Here's how the part is built. I have some questions about the finished solid (model axes, mm). Face numbers are marked on the shaded views. A direction names the side the tool comes from. Coordinates: 2 decimals unless noted, no trailing zeros. Order: outer loops, then holes, each group sorted by start corner. A loop starts at its lowest first (then second) coordinate and runs counter-clockwise, first axis right, second up.
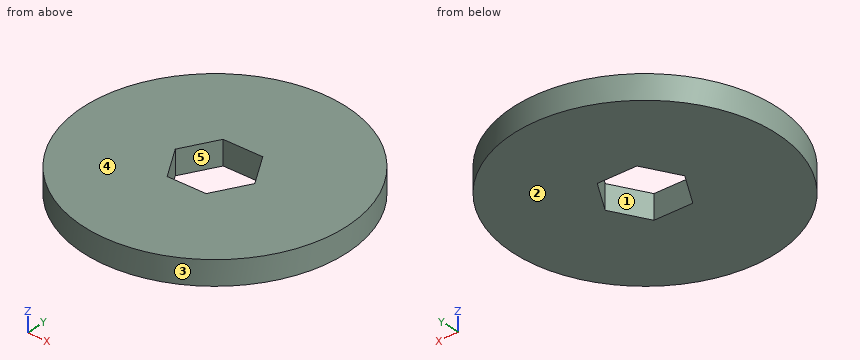
Autodesk Inventor part; units mm, degrees
ref_plane "YZ Plane" through (0, 0, 0) normal (1, 0, 0) x (0, 1, 0)
ref_plane "XZ Plane" through (0, 0, 0) normal (0, 1, 0) x (-1, 0, 0)
ref_plane "XY Plane" through (0, 0, 0) normal (0, 0, 1) x (1, 0, 0)
sketch "Sketch1" plane through (0, 0, 0) normal (0, 0, 1) x (1, 0, 0)
  line L0 (3.6662, 6.35) -> (7.3323, 0)
  line L1 (7.3323, 0) -> (3.6662, -6.35)
  line L2 (3.6662, -6.35) -> (-3.6662, -6.35)
  line L3 (-3.6662, -6.35) -> (-7.3323, 0)
  line L4 (-7.3323, 0) -> (-3.6662, 6.35)
  line L5 (-3.6662, 6.35) -> (3.6662, 6.35)
  circle A0 centre (0, 0) radius 25.273
  circle A1 centre (0, 0) radius 7.3323 construction
  dimension "d0" = 12.7
  dimension "d2" = 50.546
  dimension "d3" = 17.9407
extrude "Extrusion1" add sketch "Sketch1" against normal blind 4.7625
thicken "Reduce Outside Diameter" operation add thickness 0.127 both sides no extend neighbours yes toward (-0.9967573, 0.0804666, 0) faces at (25.191, -2.0336, -3.175)
thicken "Thicken2" operation add thickness 0.127 both sides no extend neighbours yes toward (-0.8660254, -0.5, 0) faces at (-4.8882, -4.2333, -1.5875) (-6.1103, 2.1167, -1.5875) (-1.2221, 6.35, -1.5875) (4.8882, 4.2333, -1.5875) (11.0881, 6.012, 0) (1.2221, -6.35, -1.5875)
equation "\"d0\" = hexSize"
equation "\"d2\" = externalDiameter - 2 * printSpacing"
equation "\"d4\" = thickness"
equation "\"d6\" = printSpacing"
equation "\"d7\" = printSpacing"
equation "\"d8\" = printSpacing"
equation "\"d9\" = printSpacing"
equation "\"hexSize\" = 12.7"
equation "\"externalDiameter\" = 50.8"
equation "\"thickness\" = 4.7625"
equation "\"printSpacing\" = 0.127"
properties part number "1_2x2x3_16-hexBearing" material "PC/ABS Plastic"
Q1. If we section it at C-C on x = -5.5: Write out the boundary of the cut face in (y, z), then the cut area to 3 significant figures.
Q2. I need wall thicknesses on L1, parallel to X at y = -5, z = -3; L2, parallel to Y at x = 1, z = -3.3; L3, parallel to Y at x = 5.5, z = -3.7. Which ranges of each line are inside material? Lowest first, please.
Q3. Will this pin go through, and if not, where does the flat tip stop? pin 1 (2 mm diameter, centred on x = 7.5, z = -3.5, fed in from +Y).
Q4. For the marked faces 4 and 5, which set-ups out of +Z, -Z, +X, -X, +Y, -Y let a thin tool reach every point of the face, with its end or its side?
Q5. If we section it at B-B on z = -3.15: Write out the boundary of the cut face in (x, y), then the cut area to 3 significant figures.
Q6. If we section it at D-D on y = 12: Write out the boundary of the cut face in (x, z).
Q7. If we section it at A-A on x = 0: Write out the boundary of the cut face in (y, z).
Q8. We'd pull the mould along Y, two halves only. Please class the marked faces 1, 2 and 3: pulls with the +Y half, pulls with the -Y half, needs draft (parallel to the pull), parting line crosses it, or undercut.
Reply:
1. outline: (-24.54, -4.76) - (-3.43, -4.76) - (-3.43, -0.13) - (-24.54, -0.13) - close; (3.43, -4.76) - (24.54, -4.76) - (24.54, -0.13) - (3.43, -0.13) - close
1. area: 196 mm2
2. L1: x = -24.64 to -4.59, 4.45 to 24.64
2. L2: y = -25.13 to -6.48, 6.48 to 25.13
2. L3: y = -24.54 to -3.17, 3.43 to 24.54
3. pin 1: stops at y = 24.29
4. face 4: +Z, +X, -X, +Y, -Y
4. face 5: +Z, -Z
5. outline: circle Ø50.29 at (0, 0); hole (-7.48, 0) - (-3.74, -6.48) - (3.59, -6.48) - (7.41, 0.13) - (3.74, 6.48) - (-3.74, 6.48) - close
5. area: 1,840 mm2
6. outline: (-22.1, -4.76) - (22.1, -4.76) - (22.1, -0.13) - (-22.1, -0.13) - close
7. outline: (-25.15, -4.76) - (-6.48, -4.76) - (-6.48, -0.13) - (-25.15, -0.13) - close; (6.48, -4.76) - (25.15, -4.76) - (25.15, -0.13) - (6.48, -0.13) - close
8. face 1: undercut
8. face 2: needs draft
8. face 3: parting line crosses it
